Could you check a few things on this model? Use its own coordinates, in mm. Face numbers are marked on the shaded views. A direction names the side the tool comes from. Round coordinates to 2 decimals unless told otherwise and drop trailing zeros. Write each loop counter-clockwise with the first axis right and the second up, starting at its lowest first coordinate (ties: lowest second). Pieces come first, ordered by that corner, then holes. Notation, with made-up numbers: (-20.75, 48.25) -> (-2.75, 48.25) arc R27 ccw to (-2.75, 78.25) -> close; hole circle Ø6 at (67.5, -18.5). An arc over 180 degrees is marked (long way). Return JSON: item names as keys, results as strings.
from build123d import *

# Parameters (mm, degrees)
SKETCH1_W           = 203.2
SKETCH1_H           = 152.4
BOSS_EXTRUDE1_DEPTH = 6.35
SKETCH2_W           = 203.2
SKETCH2_H           = 152.4
SKETCH2_W_2         = 190.5
SKETCH2_H_2         = 139.7
BOSS_EXTRUDE2_DEPTH = 76.2
SKETCH3_W           = 203.2
SKETCH3_H           = 152.4
SKETCH3_W_2         = 196.85
SKETCH3_H_2         = 146.05
BOSS_EXTRUDE3_DEPTH = 6.35


with BuildPart() as part:
    # Sketch1 → Boss-Extrude1 (new body)
    with BuildSketch(Plane(origin=(0, 0, 0), x_dir=(1, 0, 0), z_dir=(0, 1, 0))):
        Rectangle(SKETCH1_W, SKETCH1_H)
    extrude(amount=BOSS_EXTRUDE1_DEPTH)

    # Sketch2 → Boss-Extrude2 (add)
    with BuildSketch(Plane(origin=(0, 6.35, 0), x_dir=(1, 0, 0), z_dir=(0, 1, 0))):
        Rectangle(SKETCH2_W, SKETCH2_H)
        Rectangle(SKETCH2_W_2, SKETCH2_H_2, mode=Mode.SUBTRACT)
    extrude(amount=BOSS_EXTRUDE2_DEPTH)

    # Sketch3 → Boss-Extrude3 (add)
    with BuildSketch(Plane(origin=(0, 82.55, 0), x_dir=(1, 0, 0), z_dir=(0, 1, 0))):
        Rectangle(SKETCH3_W, SKETCH3_H)
        Rectangle(SKETCH3_W_2, SKETCH3_H_2, mode=Mode.SUBTRACT)
    extrude(amount=BOSS_EXTRUDE3_DEPTH)


solid = part.part
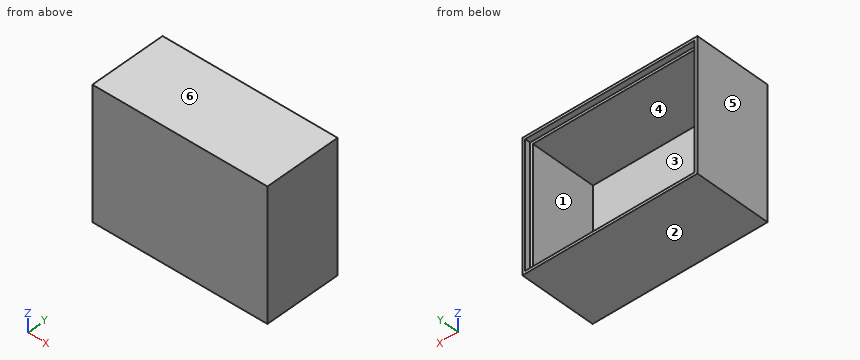
1) I want a section at C-C, the plane z = 61. Please give me the cut outline in (x, y) (3 decimals), and give its area (3 significant figures).
Return value:
{"outline": "(-101.6, 0) -> (101.6, 0) -> (101.6, 88.9) -> (98.425, 88.9) -> (98.425, 82.55) -> (95.25, 82.55) -> (95.25, 6.35) -> (-95.25, 6.35) -> (-95.25, 82.55) -> (-98.425, 82.55) -> (-98.425, 88.9) -> (-101.6, 88.9) -> close", "area": "2,300 mm²"}
2) If I drill on probe 1 along X at (y, z) = (80.5, -65); probe 2 along Z at (x, y) = (-78, 50.5); probe 3 along Z at (x, y) = (-41.5, 84.5) (3 decimals), over which ranges is the centre line in solid material (lowest first)? Write a range as [from, to].
Return value:
{"probe 1": "[-101.6, -95.25], [95.25, 101.6]", "probe 2": "[-76.2, -69.85], [69.85, 76.2]", "probe 3": "[-76.2, -73.025], [73.025, 76.2]"}
3) I want a section at A-A, the plane x = -4.5. Please give me the cut outline in (y, z) (3 decimals), and give its area (3 significant figures).
Return value:
{"outline": "(0, -76.2) -> (88.9, -76.2) -> (88.9, -73.025) -> (82.55, -73.025) -> (82.55, -69.85) -> (6.35, -69.85) -> (6.35, 69.85) -> (82.55, 69.85) -> (82.55, 73.025) -> (88.9, 73.025) -> (88.9, 76.2) -> (0, 76.2) -> close", "area": "1,980 mm²"}
4) For the marked faces 1 and 2, which set-ups out of +Z, -Z, +X, -X, +Y, -Y let a thin tool reach every point of the face, with its end or its side?
Return value:
{"face 1": "+Y", "face 2": "-Z, +X, -X, +Y, -Y"}
5) Will this pin go through, and if not, where does the flat tip stop? pin 1 Ø8 at (x, z) = (-12.5, 36) entering from +Y.
Return value:
{"pin 1": "y = 6.35"}
6) I want a section at B-B, the plane y = 67. Please give me the cut outline in (x, z).
Return value:
{"outline": "(-101.6, -76.2) -> (101.6, -76.2) -> (101.6, 76.2) -> (-101.6, 76.2) -> close; hole (-95.25, -69.85) -> (95.25, -69.85) -> (95.25, 69.85) -> (-95.25, 69.85) -> close"}
7) Thinking about a two-plate mould opening in Z: for the marked faces 3, 4, 5 and 6, which applies, pulls with the +Z half, pulls with the -Z half, needs draft (parallel to the pull), parting line crosses it, or undercut?
Return value:
{"face 3": "undercut", "face 4": "undercut", "face 5": "needs draft", "face 6": "pulls with the +Z half"}
